Autodesk Inventor part; units mm, degrees
ref_plane "YZ Plane" through (0, 0, 0) normal (1, 0, 0) x (0, 1, 0)
ref_plane "XZ Plane" through (0, 0, 0) normal (0, 1, 0) x (-1, 0, 0)
ref_plane "XY Plane" through (0, 0, 0) normal (0, 0, 1) x (1, 0, 0)
sketch "Esquisse1" plane through (0, 0, 0) normal (0, 0, 1) x (1, 0, 0)
  line L0 (-9.5, 14.5) -> (9.5, 14.5)
  line L1 (9.5, 14.5) -> (9.5, -14.5)
  line L2 (9.5, -14.5) -> (-9.5, -14.5)
  line L3 (-9.5, -14.5) -> (-9.5, 14.5)
  line L4 (-13.3, 0) -> (13.3, 0)
  line L5 (0, -20.3) -> (0, 20.3)
  circle A0 centre (0, 12.5) radius 1
  point P0 (0, 0)
  dimension "d0" = 19
  dimension "d1" = 29
  dimension "d2" = 2
  dimension "d3" = 2
extrude "Extrusion1" add sketch "Esquisse1" along normal blind 2 contours L0 L5 A0 L4 L3 | L0 L1 L4 L5 A0 | L4 L5 L2 L3 | L4 L1 L2 L5
sketch "Esquisse2" plane through (0, 0, 0) normal (0, 0, -1) x (-1, 0, 0)
  line L0 (-4, -12) -> (4, -12)
  line L1 (4, -12) -> (4, -17)
  line L2 (4, -17) -> (-4, -17)
  line L3 (-4, -17) -> (-4, -12)
  line L4 (0, -23.3) -> (0, 20.8)
  line L5 (9.5, -14.5) -> (-9.5, -14.5)
  point P0 (0, 0)
  dimension "d6" = 8
  dimension "d7" = 5
  dimension "d8" = 2.5
extrude "Extrusion2" add sketch "Esquisse2" along normal mid plane 1.25
chamfer "Chanfrein1" distance 0.5 angle 45 3 edges at (0, -12, -0.625) (4, -14.5, -0.625) (-4, -14.5, -0.625)
extrude "Extrusion3" add sketch "Esquisse1" against normal blind 4 contours A0 L5 | L5 A0
sketch "Esquisse3" plane through (0, 12.5, -4) normal (0, 0, -1) x (-1, 0, 0)
  arc A0 (0, -1.25) -> (0, 1.25) centre (0, 0) ccw
  line L0 (0, 1.25) -> (0, -1.25)
  line L1 (0.25, 1.3454) -> (0.25, -1.2696)
  line L2 (-0.25, 1.3454) -> (-0.25, -1.2696)
  line L3 (-0.25, 1.3454) -> (0.25, 1.3454)
  line L4 (0.25, -1.2696) -> (-0.25, -1.2696)
  line L5 (-0.9682, 0.25) -> (0.9682, 0.25)
  circle A1 centre (0, 0) radius 1
  line L6 (-0.9015, -0.25) -> (1.035, -0.25)
  circle A2 centre (0, 0) radius 1
  line L7 (-0.9682, 0.25) -> (-1.0579, 0.25)
  line L8 (-1.0579, -0.25) -> (-0.9015, -0.25)
  line L9 (1.035, 0.25) -> (0.9682, 0.25)
  line L10 (1.035, 0.25) -> (1.2927, 0.25)
  line L11 (1.2927, 0.25) -> (1.2927, -0.25)
  line L12 (1.2927, -0.25) -> (1.035, -0.25)
  line L13 (-1.0579, 0.25) -> (-1.4678, 0.25)
  line L14 (-1.4678, 0.25) -> (-1.4678, -0.25)
  line L15 (-1.4678, -0.25) -> (-1.0579, -0.25)
  point P0 (0, -12.5)
  point P1 (0, 0)
  point P2 (0.25, 0.25)
  point P3 (-0.25, 0.25)
  point P4 (-0.25, -0.25)
  point P5 (0.25, -0.25)
  point P6 (0, 1.2247)
  point P7 (0, -1.2247)
  point P8 (1.2247, 0.25)
  point P9 (0.25, 1.2247)
  point P10 (1.2247, -0.25)
  point P11 (0.25, -1.2247)
  point P12 (0, -0.25)
  point P13 (0, 0.25)
  dimension "d16" = 1.25
  dimension "d17" = 0
  dimension "d18" = 0
  dimension "d19" = 13.75
  dimension "d21" = 0.25
  dimension "d22" = 0.25
  dimension "d56" = 1.0427
  dimension "d57" = 2.7604
  dimension "d58" = 0.5
  dimension "d59" = 1.0954
  dimension "d60" = 1.5196
  dimension "d61" = 0.2577
  dimension "d62" = 0.2577
  dimension "d63" = 1.0427
  dimension "d64" = 1.0427
  dimension "d65" = 1.0954
  dimension "d66" = 1.0427
  dimension "d67" = 0.5
  dimension "d68" = 1.0427
  dimension "d69" = 0
  dimension "d70" = 1.2927
  dimension "d71" = 0.9747
  dimension "d72" = 1.2927
  dimension "d73" = 1.4747
  dimension "d74" = 1.5427
  dimension "d75" = 0
  dimension "d76" = 1.5427
  dimension "d77" = 0.5
  dimension "d78" = 2.3506
  dimension "d79" = 2.3506
revolve "Révolution1" add sketch "Esquisse3" angle 360 about axis through (0, 13.75, -4) along (0, -1, 0) contours L0 A1 L1 A0 | L1 A1 L6 L12 A0 | L0 L6 L1 A1 | L12 L6 A1 L9 L10 A0 | L1 L6 A1 | L0 L5 L1 L6 | L10 L9 A1 L1 A0 | L1 L5 A1 L6 | L0 A1 L1 L5 | L1 A1 L0 A0 | L1 A1 L5
extrude "Extrusion6" cut sketch "Esquisse3" along normal blind 4 and the other way blind 3 contours L0 A1 L1 A0 | A0 L1 L4 L2 A1 L0 | A1 L2 L6 L0 | L0 L6 L1 A1 | L12 L6 A1 L9 L10 A0 | A0 L10 L11 L12 | L6 L2 L5 L0 | L0 L5 L1 L6 | L1 L5 A1 L6 | L5 L2 A1 L0 | L0 A1 L1 L5 | L6 L8 A1 L5 L2 | L8 L15 L14 L13 L7 A1 | L1 A1 L0 A0 | A0 L0 A1 L2 L3 L1
sketch "Esquisse4" plane through (0, 12.5, 0) normal (0, 0, 1) x (1, 0, 0)
  circle A0 centre (0, 0) radius 1
  point P0 (0, -12.5)
extrude "Extrusion7" add sketch "Esquisse4" along normal blind 2
sketch "Esquisse5" plane through (-9.5, 14.5, 0) normal (0, 1, 0) x (1, 0, 0)
  line L0 (19, -2) -> (0, -2)
  line L1 (14.5, -2) -> (4.5, -2)
  line L2 (4.5, -2) -> (4.5, -1)
  line L3 (4.5, -1) -> (14.5, -1)
  line L4 (14.5, -1) -> (14.5, -2)
  line L5 (19, 0) -> (19, -2)
  point P0 (9.5, 0)
  point P1 (14.5, -1.5)
  dimension "d86" = 10
  dimension "d87" = 4.5
  dimension "d88" = 1
extrude "Extrusion8" cut sketch "Esquisse5" against normal blind 2
sketch "Esquisse6" plane through (-9.5, 12.5, 0) normal (0, 1, 0) x (1, 0, 0)
  line L0 (4.5, -2) -> (4.5, -1)
  line L1 (14.5, -1) -> (14.5, -2)
  line L2 (4.5, -1) -> (14.5, -1)
  line L3 (14.5, -1) -> (14.5, -1.6)
  line L4 (14.5, -1.6) -> (4.5, -1.6)
  line L5 (4.5, -1.6) -> (4.5, -1)
  point P0 (9.5, 0)
  dimension "d91" = 0.6
extrude "Extrusion9" cut sketch "Esquisse6" against normal blind 2
properties part number "trappe"
Geometry: final body of the model. Coordinates: model frame, mm. A direction names the side the tool comes from. Round coordinates to 2 decimals unless told otherwise and drop trailing zeros. Write each loop counter-clockwise with the first axis right and the second up, starting at its lowest first coordinate (ties: lowest second). Pieces come first, ordered by that corner, then holes.
Item 1: Section query A-A (y = -13.5). Return loops of the section in (x, z) (3 decimals).
Item 2: Set-up query: faces 1 (the face through (5, 13, 1.4)), 2 (the face through (-0.7, 12.75, -3.1)), 3 (the face through (0, -16, 0.625)), 4 (the face through (-0.25, 13, -3)). Return all of +Z, -Z, +X, -X, +Y, -Y with unobstructed straight access to the full face (end or side cutting, diameter ignored); none if empty.
Item 3: Material intervals for L1, parallel to Z at x = 4.25, y = -13; L2, parallel to Z at x = -1.5, y = 12; L3, parallel to Z at x = 0.5, y = 13.5, sorted ascending.
Item 4: Pin query (flat end, axial travel): P1, Ø0.8, axis at x = -0.5, z = -4, coming from the +Y side; P2, Ø0.5, axis at x = -1, z = -3.5, coming from the -Y side; P3, Ø4, axis at x = -6, y = 5.5, coming from the -Z side. Return the tip coordinate at first contact, or that it passes through.
Item 5: Mould query, pull axis Z, two halves, no side actions, for faces 5 (the face through (-0.25, 12, -3)), 6 (the face through (0, 13, -1)), 7 (the face through (0, 12, 1.6)). Classes: +Z half, -Z half, draft (parallel to the pull), parting line (faces both ways), or undercut.
Item 6: Section query B-B (z = -1.5). Return loops of the section in (x, y), plus the area to 3 significant figures.
Item 7: Section query D-D (y = -3.5). Return loops of the section in (x, z).
Item 8: Section query C-C (x = 6.5). Return loops of the section in (y, z).
Completed:
1. outline: (-9.5, 0) - (-4, 0) - (-4, -0.125) - (-3.5, -0.625) - (3.5, -0.625) - (4, -0.125) - (4, 0) - (9.5, 0) - (9.5, 2) - (-9.5, 2) - close
2. face 1: +Y
2. face 2: -Z, +X, -X
2. face 3: +Z, +X, -X, -Y
2. face 4: -Z, +Y, -Y
3. L1: z = 0 to 2
3. L2: z = 0 to 1, 1.6 to 2
3. L3: z = -4.56 to -3.44, 0 to 1
4. P1: stops at y = 13.72
4. P2: stops at y = 11.6
4. P3: stops at z = 0
5. face 5: draft
5. face 6: -Z half
5. face 7: undercut
6. outline: (-0.97, 12.25) arc R1 ccw to (-0.25, 11.53) - (-0.25, 12.25) - close; (-0.97, 12.75) - (-0.25, 12.75) - (-0.25, 13.47) arc R1 ccw to start; (0.25, 11.53) arc R1 ccw to (0.97, 12.25) - (0.25, 12.25) - close; (0.25, 12.75) - (0.97, 12.75) arc R1 ccw to (0.25, 13.47) - close
6. area: 1.41 mm2
7. outline: (-9.5, 0) - (9.5, 0) - (9.5, 2) - (-9.5, 2) - close
8. outline: (-14.5, 0) - (14.5, 0) - (14.5, 2) - (-14.5, 2) - close
